The listing builds one solid part. Answer for the finished solid, in the listing's coordinates (mm). Coordinates: 2 decimals unless noted, no trailing zeros. Loops run counter-clockwise (first coordinate to the right, second up) from the corner with the lowest first, then second, coordinate; pieces in that order, holes last. Notation, with made-up numbers: (78.25, -21.75) -> (122.25, -21.75) arc R7 ccw to (122.25, -12.75) -> close; hole circle Ø6 at (-11.5, -37.75). An arc over 180 degrees is marked (long way). Answer in a Markdown table with one row per item.
```python
from build123d import *

# Parameters (mm, degrees)
BOSS_EXTRUDE1_DEPTH = 500
CHAMFER1_SIZE       = 0.2
LPATTERN1_COUNT     = 20
LPATTERN1_PITCH     = 25


with BuildPart() as part:
    # Sketch1 → Boss-Extrude1 (new body)
    with BuildSketch(Plane.XY):
        with BuildLine():
            Line((12.21524152, 8.978261926), (12.21524152, 7.53727892))
            ThreePointArc((12.21524152, 7.53727892), (11.921348894, 7.453790184), (11.71524152, 7.228261926))
            Line((11.71524152, 7.228261926), (11.21524152, 7.228261926))
            Line((11.21524152, 7.228261926), (11.21524152, 6.728261926))
            Line((11.21524152, 6.728261926), (11.71524152, 6.728261926))
            ThreePointArc((11.71524152, 6.728261926), (11.921348894, 6.502733668), (12.21524152, 6.419244931))
            Line((12.21524152, 6.419244931), (12.21524152, 1.278261926))
            Line((12.21524152, 1.278261926), (11.91524152, 0.978261926))
            Line((11.91524152, 0.978261926), (0.51524152, 0.978261926))
            Line((0.51524152, 0.978261926), (0.21524152, 1.278261926))
            Line((0.21524152, 1.278261926), (0.21524152, 6.419244931))
            ThreePointArc((0.21524152, 6.419244931), (0.509134147, 6.502733668), (0.71524152, 6.728261926))
            Line((0.71524152, 6.728261926), (1.21524152, 6.728261926))
            Line((1.21524152, 6.728261926), (1.21524152, 7.228261926))
            Line((1.21524152, 7.228261926), (0.71524152, 7.228261926))
            ThreePointArc((0.71524152, 7.228261926), (0.509134147, 7.453790184), (0.21524152, 7.53727892))
            Line((0.21524152, 7.53727892), (0.21524152, 8.978261926))
            Line((0.21524152, 8.978261926), (12.21524152, 8.978261926))
        make_face()
    extrude(amount=-BOSS_EXTRUDE1_DEPTH)

    # Chamfer1
    chamfer1_edges = [part.edges().sort_by_distance(p)[0] for p in [
        (0.509134147, 7.453790184, -500),
        (0.96524152, 7.228261926, -500),
        (12.21524152, 8.257770423, 0),
        (1.21524152, 6.978261926, -500),
        (11.921348894, 7.453790184, 0),
        (11.46524152, 7.228261926, 0),
        (11.21524152, 6.978261926, 0),
        (11.46524152, 6.728261926, 0),
        (11.921348894, 6.502733668, 0),
        (12.21524152, 3.848753429, 0),
        (12.06524152, 1.128261926, 0),
        (6.21524152, 0.978261926, 0),
        (0.96524152, 6.728261926, -500),
        (0.36524152, 1.128261926, 0),
        (0.21524152, 3.848753429, 0),
        (0.509134147, 6.502733668, 0),
        (0.96524152, 6.728261926, 0),
        (1.21524152, 6.978261926, 0),
        (0.96524152, 7.228261926, 0),
        (0.509134147, 7.453790184, 0),
        (0.509134147, 6.502733668, -500),
        (0.21524152, 8.257770423, 0),
        (6.21524152, 8.978261926, 0),
        (0.21524152, 3.848753429, -500),
        (0.36524152, 1.128261926, -500),
        (6.21524152, 0.978261926, -500),
        (12.06524152, 1.128261926, -500),
        (12.21524152, 3.848753429, -500),
        (6.21524152, 8.978261926, -500),
        (11.921348894, 6.502733668, -500),
        (11.46524152, 6.728261926, -500),
        (11.21524152, 6.978261926, -500),
        (11.46524152, 7.228261926, -500),
        (11.921348894, 7.453790184, -500),
        (12.21524152, 8.257770423, -500),
        (0.21524152, 8.257770423, -500),
    ]]
    chamfer(chamfer1_edges, length=CHAMFER1_SIZE)

    # Sketch3 → CBORE for M4 Hex Head Machine Screw1 (revolve, cut)
    with BuildSketch(Plane(origin=(6.21524152, 8.978261926, -12.5), x_dir=(0, 0, 1), z_dir=(1, 0, 0))):
        Polygon((0, 0), (0, 8), (2.25, 8), (2.25, 4.5), (4, 4.5), (4, 0.25), (4.25, 0), align=None)
    cbore_for_m4_hex_head_machine_screw1 = revolve(axis=Axis((6.21524152, 15.328261926, -12.5), (0, -1, 0)), mode=Mode.SUBTRACT)

    # LPattern1: CBORE for M4 Hex Head Machine Screw1 ×20
    with Locations(*[(0, 0, -i * LPATTERN1_PITCH) for i in range(1, LPATTERN1_COUNT)]):
        add(cbore_for_m4_hex_head_machine_screw1, mode=Mode.SUBTRACT)


solid = part.part
```
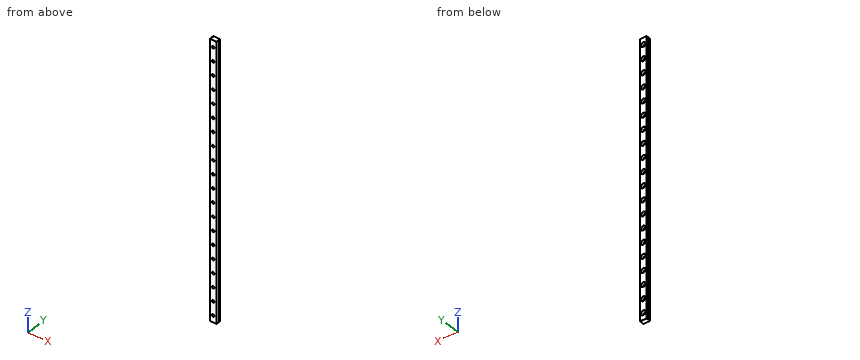
Item 1: A flat-ended cylindrical pin translates along its axis: pin 1 Ø5 at (x, z) = (6.22, -462.5) entering from +Y. Find the tip coordinate at first contact, or state that the pin passes through.
Findings below:
| item | result |
|---|---|
| pin 1 | stops at y = 4.48 |
Item 2: Find the intervals of material crossed by probe 1 along X at (y, z) = (2.2, -362.5); probe 2 along Y at (x, z) = (11.5, -383.5); probe 3 along X at (y, z) = (7.4, -212.5), in increasing order.
Findings below:
| item | result |
|---|---|
| probe 1 | x = 0.22 to 3.97, 8.47 to 12.22 |
| probe 2 | y = 0.98 to 6.73, 7.23 to 8.98 |
| probe 3 | x = 0.58 to 2.22, 10.22 to 11.85 |
Item 3: A cutting plane is placed at A-A, the plane z = -49. Determine the outline of the cut face in (x, y), plus the area to 3 significant figures.
Findings below:
| item | result |
|---|---|
| outline | (0.22, 1.28) -> (0.52, 0.98) -> (11.92, 0.98) -> (12.22, 1.28) -> (12.22, 6.42) arc R0.56 cw to (11.72, 6.73) -> (11.22, 6.73) -> (11.22, 7.23) -> (11.72, 7.23) arc R0.56 cw to (12.22, 7.54) -> (12.22, 8.98) -> (0.22, 8.98) -> (0.22, 7.54) arc R0.56 cw to (0.72, 7.23) -> (1.22, 7.23) -> (1.22, 6.73) -> (0.72, 6.73) arc R0.56 cw to (0.22, 6.42) -> close |
| area | 94.5 mm2 |
Item 4: A cutting plane is placed at B-B, the plane y = 2.75. Count the separate pieces of the cut face and the enclosed holes in it, plus the area to 3 significant figures.
Findings below:
| item | result |
|---|---|
| separate pieces | 1 |
| enclosed holes | 20 |
| area | 5,680 mm2 |
